Could you check a few things on this model? Use its own coordinates, in mm. A direction names the side the tool comes from. Coordinates: 2 decimals unless noted, no trailing zeros. Write each loop counter-clockwise with the first axis right and the second up, starting at its lowest first coordinate (ties: lowest second). Pieces come first, ordered by that corner, then holes.
Item 1: Thinking about a two-plate mould opening in X: for faces 3 (the flat face through (12.5, 0, 1)), 4 (the flat face through (10.25, 0, 1)), 5 (the flat face through (0, -24.9, 1)), which applies, +X half, -X half, draft (parallel to the pull), parting line (faces both ways), or undercut?
Item 2: I want a section at B-B on x = 1.75. Please give me the cut outline in (y, z).
Item 3: If I drill on probe 1 along Y at (x, z) = (6, 2.15); probe 2 along X at (y, z) = (-1.5, 2.4), over which ranges is the centre line in solid material (lowest first)?
Item 4: I want a section at C-C on z = 1. Please give me the cut outline in (x, y).
Item 5: I want a section at A-A on y = 3. Please give me the cut outline in (x, z).
Item 6: Which directions (+Z, -Z, +X, -X, +Y, -Y) give clear straight access to the entire face, cutting with the end or side of a thin tool? Please do faces 1 (the flat face through (-10.25, 0, 1)), 2 (the flat face through (-12.5, 0, 1)).
Autodesk Inventor part; units mm, degrees
ref_plane "YZ Plane" through (0, 0, 0) normal (1, 0, 0) x (0, 1, 0)
ref_plane "XZ Plane" through (0, 0, 0) normal (0, 1, 0) x (-1, 0, 0)
ref_plane "XY Plane" through (0, 0, 0) normal (0, 0, 1) x (1, 0, 0)
sketch "Sketch1" plane through (0, 0, 0) normal (0, 0, 1) x (1, 0, 0)
  line L0 (-17.5, 0) -> (17.5, 0) construction
  line L1 (0, -34.86) -> (0, 34.86) construction
  line L2 (-12.5, 24.9) -> (12.5, 24.9)
  line L3 (12.5, 24.9) -> (12.5, -24.9)
  line L4 (12.5, -24.9) -> (-12.5, -24.9)
  line L5 (-12.5, -24.9) -> (-12.5, 24.9)
  line L6 (-10.25, 21.75) -> (10.25, 21.75)
  line L7 (10.25, 21.75) -> (10.25, -21.75)
  line L8 (10.25, -21.75) -> (-10.25, -21.75)
  line L9 (-10.25, -21.75) -> (-10.25, 21.75)
  point P0 (0, 0)
  dimension "d0" = 20.5
  dimension "d1" = 25
  dimension "d2" = 49.8
  dimension "d3" = 43.5
extrude "Extrusion1" add sketch "Sketch1" along normal blind 3
properties part number "20_Cube_Insert_Sample_clamp"
Response values:
1. face 3: +X half
1. face 4: undercut
1. face 5: draft
2. outline: (-24.9, 0) - (-21.75, 0) - (-21.75, 3) - (-24.9, 3) - close; (21.75, 0) - (24.9, 0) - (24.9, 3) - (21.75, 3) - close
3. probe 1: y = -24.9 to -21.75, 21.75 to 24.9
3. probe 2: x = -12.5 to -10.25, 10.25 to 12.5
4. outline: (-12.5, -24.9) - (12.5, -24.9) - (12.5, 24.9) - (-12.5, 24.9) - close; hole (-10.25, -21.75) - (10.25, -21.75) - (10.25, 21.75) - (-10.25, 21.75) - close
5. outline: (-12.5, 0) - (-10.25, 0) - (-10.25, 3) - (-12.5, 3) - close; (10.25, 0) - (12.5, 0) - (12.5, 3) - (10.25, 3) - close
6. face 1: +Z, -Z
6. face 2: +Z, -Z, -X, +Y, -Y
